```python
from build123d import *

# Parameters (mm, degrees)
SKETCH1_W           = 25.4
SKETCH1_H           = 25.4
BOSS_EXTRUDE1_DEPTH = 355.6
FILLET1_R           = 1.5875
HOLE1_OUTLINE_R     = 2.5527
HOLE1_DEPTH         = 355.6
SKETCH7_W           = 6.5278
SKETCH7_H           = 2.2352
CUT_EXTRUDE2_DEPTH  = 355.6
FILLET4_R           = 0.396875
CIRPATTERN2_DEPTH   = 355.6


# Read off the part's stored shape, not the designer's step: Hole1, CirPattern2
with BuildPart() as part:
    # Sketch1 → Boss-Extrude1 (new body)
    with BuildSketch(Plane.XY):
        Rectangle(SKETCH1_W, SKETCH1_H)
    extrude(amount=BOSS_EXTRUDE1_DEPTH)

    # Fillet1
    fillet1_edges = [part.edges().sort_by_distance(p)[0] for p in [
        (12.7, -12.7, 177.8),
        (-12.7, -12.7, 177.8),
        (-12.7, 12.7, 177.8),
        (12.7, 12.7, 177.8),
    ]]
    fillet(fillet1_edges, radius=FILLET1_R)

    # Hole1 outline → Hole1 (cut)
    with BuildSketch(Plane.XY):
        with Locations((0, -0.048792482)):
            Circle(HOLE1_OUTLINE_R)
    extrude(amount=HOLE1_DEPTH, mode=Mode.SUBTRACT)

    # Sketch7 → Cut-Extrude2 (cut)
    with BuildSketch(Plane.XY.offset(355.6)):
        with Locations((0, 11.5824)):
            Rectangle(SKETCH7_W, SKETCH7_H)
        Polygon((-3.175, 4.5212), (-7.3025, 10.4648), (7.3025, 10.4648), (3.175, 4.5212), align=None)
    extrude(amount=-CUT_EXTRUDE2_DEPTH, mode=Mode.SUBTRACT)

    # Fillet4
    fillet4_edges = [part.edges().sort_by_distance(p)[0] for p in [
        (-3.2639, 10.4648, 177.8),
        (-3.2639, 12.7, 177.8),
        (3.2639, 12.7, 177.8),
        (3.2639, 10.4648, 177.8),
    ]]
    fillet(fillet4_edges, radius=FILLET4_R)

    # CirPattern2 outline → CirPattern2 (cut)
    with BuildSketch(Plane.XY):
        with BuildLine():
            ThreePointArc((-3.660775, -10.562384964), (-3.380141996, -10.67862696), (-3.2639, -10.959259964))
            Line((-3.2639, -10.959259964), (-3.2639, -12.7))
            Line((-3.2639, -12.7), (3.2639, -12.7))
            Line((3.2639, -12.7), (3.2639, -10.959259964))
            ThreePointArc((3.2639, -10.959259964), (3.380141996, -10.67862696), (3.660775, -10.562384964))
            Line((3.660775, -10.562384964), (7.3025, -10.562384964))
            Line((7.3025, -10.562384964), (3.175, -4.618784964))
            Line((3.175, -4.618784964), (-3.175, -4.618784964))
            Line((-3.175, -4.618784964), (-7.3025, -10.562384964))
            Line((-7.3025, -10.562384964), (-3.660775, -10.562384964))
        make_face()
        with BuildLine():
            Line((-12.7, -3.312692482), (-10.910467482, -3.312692482))
            ThreePointArc((-10.910467482, -3.312692482), (-10.629834478, -3.428934478), (-10.513592482, -3.709567482))
            Line((-10.513592482, -3.709567482), (-10.513592482, -7.351292482))
            Line((-10.513592482, -7.351292482), (-4.569992482, -3.223792482))
            Line((-4.569992482, -3.223792482), (-4.569992482, 3.126207518))
            Line((-4.569992482, 3.126207518), (-10.513592482, 7.253707518))
            Line((-10.513592482, 7.253707518), (-10.513592482, 3.611982518))
            ThreePointArc((-10.513592482, 3.611982518), (-10.629834478, 3.331349514), (-10.910467482, 3.215107518))
            Line((-10.910467482, 3.215107518), (-12.7, 3.215107518))
            Line((-12.7, 3.215107518), (-12.7, -3.312692482))
        make_face()
        with BuildLine():
            ThreePointArc((10.513592482, -3.709567482), (10.629834478, -3.428934478), (10.910467482, -3.312692482))
            Line((10.910467482, -3.312692482), (12.7, -3.312692482))
            Line((12.7, -3.312692482), (12.7, 3.215107518))
            Line((12.7, 3.215107518), (10.910467482, 3.215107518))
            ThreePointArc((10.910467482, 3.215107518), (10.629834478, 3.331349514), (10.513592482, 3.611982518))
            Line((10.513592482, 3.611982518), (10.513592482, 7.253707518))
            Line((10.513592482, 7.253707518), (4.569992482, 3.126207518))
            Line((4.569992482, 3.126207518), (4.569992482, -3.223792482))
            Line((4.569992482, -3.223792482), (10.513592482, -7.351292482))
            Line((10.513592482, -7.351292482), (10.513592482, -3.709567482))
        make_face()
    extrude(amount=CIRPATTERN2_DEPTH, mode=Mode.SUBTRACT)


solid = part.part
```
Source: CAD feature listing. Evaluate the final solid. Frame: model axes, mm. A direction names the side the tool comes from. Round coordinates to 2 decimals unless told otherwise and drop trailing zeros. Use a Markdown table: item, result. Add a question column.
1. Contact query for flat-ended pins moving along their axis: pin 1 (3 mm diameter, centred on x = -0.5, z = 238.5, fed in from +Y); pin 2 (0.5 mm diameter, centred on y = -12, z = 160.5, fed in from -X); pin 3 (1.9 mm diameter, centred on y = -1, z = 256, fed in from +X). Output: stop coordinate, or through.
2. Ray query, line 1 along X through (y, z) = (-11.5, 239.5); line 2 along Y through (x, z) = (-4.75, 25); line 3 along X through (y, z) = (-3.75, 87). Return the intervals inside material, ascending. Write a range as [from, to].
3. Set-up query: faces 1 (the flat face through (0, -4.619, 175)), 2 (the flat face through (-12.7, 7, 175)), 3 (the flat face through (-4.57, 0, 175)). Return all of +Z, -Z, +X, -X, +Y, -Y with unobstructed straight access to the full face (end or side cutting, diameter ignored); none if empty.
4. Pull-direction query (X, two-part tool) for faces 4 (the flat face through (-7.5, 5.16, 175.31)), 5 (the flat face through (-7.583, -5.316, 175.311)), 6 (the flat face through (3, 0, 355.6)), 7 (the flat face through (12.7, -7, 175)); classes: +X half, -X half, draft (parallel to the pull), parting line (faces both ways), or undercut.
Solution:
| question | item | result |
|---|---|---|
| 1 | pin 1 | stops at y = 4.52 |
| 1 | pin 2 | stops at x = -12.57 |
| 1 | pin 3 | stops at x = 4.57 |
| 2 | line 1 | x = [-12.65, -3.26], [3.26, 12.65] |
| 2 | line 2 | y = [-12.7, -10.56], [-6.89, -3.35], [3.25, 6.79], [10.46, 12.7] |
| 2 | line 3 | x = [-12.7, -10.51], [-5.33, 5.33], [10.51, 12.7] |
| 3 | face 1 | +Z, -Z, -Y |
| 3 | face 2 | +Z, -Z, -X, +Y, -Y |
| 3 | face 3 | +Z, -Z, -X |
| 4 | face 4 | undercut |
| 4 | face 5 | undercut |
| 4 | face 6 | draft |
| 4 | face 7 | +X half |
